The listing builds one solid part. Answer for the finished solid, in the listing's coordinates (mm). A direction names the side the tool comes from. Give positions to 0.01 mm unless a question says otherwise; leave off trailing zeros. Loops run counter-clockwise (first coordinate to the right, second up) from the corner with the lowest first, then second, coordinate; pieces in that order, holes last.
Item 1: Section B-B, the plane y = 6 is taken. Give the vertices of the cut face in (x, z).
Item 2: Each of these flat-tipped pins is pushed along its axis until it touches: pin 1 Ø7.5 at (y, z) = (17.5, -26) entering from +X; pin 2 Ø10 at (x, y) = (-15.5, 8.5) entering from +Z; pin 3 Ø5 at (x, y) = (8, 11) entering from -Z. Where does it stop, or does it pass through?
Item 3: A tool of negligible diameter and unlimited length cuts with its end or side. For faces 1 (the face through (23, 12, -37)), 2 (the face through (-27, 13, -20)), 3 (the face through (-23, 13, -38)), 4 (the face through (-25.986, 12.775, -50.465)), from which of +Z, -Z, +X, -X, +Y, -Y can it reach the whole face along a straight path? Write none if from no direction.
Item 4: Section C-C, the plane x = -16 is taken. Give the vertices of the cut face in (y, z).
Item 5: Section D-D, the plane z = 15 is taken. Give the vertices of the cut face in (x, y), and give its area (3 significant figures).
Item 6: Consider line 1 along X through (y, z) = (9.5, -44); line 2 along X through (y, z) = (17.5, 48); line 3 along Z through (x, y) = (11, 8). Determine where each line is inside the solid, lowest interval first.
Item 7: The mould has two halves that part along Z. Classify faces 5 (the face through (-30.59, 12.32, 15.62)), 6 (the face through (-28.49, 12.32, 16.35)), 7 (the face through (34.071, 12, 45)), 8 (the face through (25, 13, -20)): pulls with the +Z half, pulls with the -Z half, needs draft (parallel to the pull), parting line crosses it, or undercut.
Item 8: Section A-A, the plane z = 32.5 is taken. Give the vertices of the cut face in (x, y), and give its area (3 significant figures).
from build123d import *

# Parameters (mm, degrees)
BOSS_EXTRU_1_DEPTH      = 25
BOSS_EXTRU_2_DEPTH      = 2
BOSS_EXTRU_3_DEPTH      = 2
BOSS_EXTRU_4_START      = -2
BOSS_EXTRU_4_DEPTH      = 2
BOSS_EXTRU_5_START      = -2
BOSS_EXTRU_5_DEPTH      = 2
ESQUISSE6_R             = 2.5
ENL_V_MAT_EXTRU_1_DEPTH = 10
ESQUISSE7_R             = 5
BOSS_EXTRU_6_DEPTH      = 2
ESQUISSE9_R             = 5
BOSS_EXTRU_8_DEPTH      = 2
ESQUISSE10_R            = 2.5
BOSS_EXTRU_9_DEPTH      = 2


with BuildPart() as part:
    # Esquisse1 → Boss.-Extru.1 (new body)
    with BuildSketch(Plane(origin=(0, 0, 0), x_dir=(1, 0, 0), z_dir=(0, 1, 0))):
        Polygon((-34.071067812, -59.102794325), (-34.071067812, -19.102794325), (-27, -12.031726513), (-27, 37.968273487), (-25, 37.968273487), (-25, -9.860153638), (25, -9.860153638), (25, 37.968273487), (27, 37.968273487), (27, -12.031726513), (34.071067812, -19.102794325), (34.071067812, -59.102794325), (32.071067812, -59.102794325), (32.071067812, -19.93122145), (25, -12.860153638), (-25, -12.860153638), (-32.071067812, -19.93122145), (-32.071067812, -59.102794325), align=None)
    extrude(amount=BOSS_EXTRU_1_DEPTH)

    # Esquisse2 → Boss.-Extru.2 (add)
    with BuildSketch(Plane(origin=(34.071067812, 0, 0), x_dir=(0, 0, -1), z_dir=(1, 0, 0))):
        with BuildLine():
            Line((-59.102794325, 0), (-19.102794325, 0))
            Line((-19.102794325, 0), (-19.102794325, 25))
            Line((-19.102794325, 25), (-59.102794325, 25))
            ThreePointArc((-59.102794325, 25), (-71.602794325, 12.5), (-59.102794325, 0))
        make_face()
    extrude(amount=-BOSS_EXTRU_2_DEPTH)

    # Esquisse3 → Boss.-Extru.3 (add)
    with BuildSketch(Plane(origin=(27, 0, 0), x_dir=(0, 0, -1), z_dir=(1, 0, 0))):
        with BuildLine():
            Line((37.968273487, 25), (37.968273487, 0))
            ThreePointArc((37.968273487, 0), (50.468273487, 12.5), (37.968273487, 25))
        make_face()
    extrude(amount=-BOSS_EXTRU_3_DEPTH)

    # Esquisse4 → Boss.-Extru.4 (add)
    with BuildSketch(Plane.ZY.offset(34.071067812).offset(BOSS_EXTRU_4_START)):
        with BuildLine():
            Line((59.102794325, 25), (59.102794325, 0))
            ThreePointArc((59.102794325, 0), (71.602794325, 12.5), (59.102794325, 25))
        make_face()
    extrude(amount=BOSS_EXTRU_4_DEPTH)

    # Esquisse5 → Boss.-Extru.5 (add)
    with BuildSketch(Plane.ZY.offset(27).offset(BOSS_EXTRU_5_START)):
        with BuildLine():
            Line((-37.968273487, 0), (-37.968273487, 25))
            ThreePointArc((-37.968273487, 25), (-50.468273487, 12.5), (-37.968273487, 0))
        make_face()
    extrude(amount=BOSS_EXTRU_5_DEPTH)

    # Esquisse6 → Enlèv. mat.-Extru.1 (cut)
    with BuildSketch(Plane.ZY.offset(34.071067812)):
        with Locations((59.102794325, 12.5)):
            Circle(ESQUISSE6_R)
    extrude(amount=-ENL_V_MAT_EXTRU_1_DEPTH, mode=Mode.SUBTRACT)

    # Esquisse7 → Boss.-Extru.6 (add)
    with BuildSketch(Plane(origin=(-25, 0, 0), x_dir=(0, 0, -1), z_dir=(1, 0, 0))):
        with Locations((37.968273487, 12.5)):
            Circle(ESQUISSE7_R)
    extrude(amount=BOSS_EXTRU_6_DEPTH)

    # Esquisse9 → Boss.-Extru.8 (add)
    with BuildSketch(Plane.ZY.offset(-25)):
        with Locations(Location((-39.433505518, 13.150947635, 0), (0, 0, 180))):
            Circle(ESQUISSE9_R)
    extrude(amount=BOSS_EXTRU_8_DEPTH)

    # Esquisse10 → Boss.-Extru.9 (add)
    with BuildSketch(Plane.ZY.offset(-23)):
        with Locations((-39.433505518, 13.150947635)):
            Circle(ESQUISSE10_R)
    extrude(amount=BOSS_EXTRU_9_DEPTH)


solid = part.part
Worked answers:
1. outline: (-34.07, 19.1) - (-27, 12.03) - (-27, -48.65) - (-25, -48.65) - (-25, 9.86) - (25, 9.86) - (25, -48.65) - (27, -48.65) - (27, 12.03) - (34.07, 19.1) - (34.07, 69.78) - (32.07, 69.78) - (32.07, 19.93) - (25, 12.86) - (-25, 12.86) - (-32.07, 19.93) - (-32.07, 69.78) - (-34.07, 69.78) - close
2. pin 1: stops at x = 27
2. pin 2: stops at z = 12.86
2. pin 3: stops at z = 9.86
3. face 1: none
3. face 2: -Z, -X, +Y, -Y
3. face 3: -Z, +Y, -Y
3. face 4: -Z, +X, -X
4. outline: (0, 9.86) - (25, 9.86) - (25, 12.86) - (0, 12.86) - close
5. outline: (-29.97, 0) - (-27.14, 0) - (-27.14, 25) - (-29.97, 25) - close; (27.14, 0) - (29.97, 0) - (29.97, 25) - (27.14, 25) - close
5. area: 141 mm2
6. line 1: x = -27 to -25, 25 to 27
6. line 2: x = -34.07 to -32.07, 32.07 to 34.07
6. line 3: z = 9.86 to 12.86
7. face 5: pulls with the -Z half
7. face 6: pulls with the +Z half
7. face 7: needs draft
7. face 8: undercut
8. outline: (-34.07, 0) - (-32.07, 0) - (-32.07, 25) - (-34.07, 25) - close; (32.07, 0) - (34.07, 0) - (34.07, 25) - (32.07, 25) - close
8. area: 100 mm2
